from build123d import *

# Parameters (mm, degrees)
SKETCH1_W           = 196
SKETCH1_H           = 90
BOSS_EXTRUDE1_DEPTH = 55
SKETCH2_W           = 45.25
SKETCH2_H           = 40.5
SKETCH2_H_2         = 84
CUT_EXTRUDE1_DEPTH  = 52


with BuildPart() as part:
    # Sketch1 → Boss-Extrude1 (new body)
    with BuildSketch(Plane(origin=(0, 0, 0), x_dir=(1, 0, 0), z_dir=(0, 1, 0))):
        Rectangle(SKETCH1_W, SKETCH1_H)
    extrude(amount=BOSS_EXTRUDE1_DEPTH)

    # Sketch2 → Cut-Extrude1 (cut)
    with BuildSketch(Plane(origin=(0, 55, 0), x_dir=(1, 0, 0), z_dir=(0, 1, 0))):
        with Locations((-72.375, 21.75)):
            Rectangle(SKETCH2_W, SKETCH2_H)
        with Locations((-72.375, -21.75)):
            Rectangle(SKETCH2_W, SKETCH2_H)
        with Locations((-24.125, 21.75)):
            Rectangle(SKETCH2_W, SKETCH2_H)
        with Locations((-24.125, -21.75)):
            Rectangle(SKETCH2_W, SKETCH2_H)
        with Locations((24.125, 21.75)):
            Rectangle(SKETCH2_W, SKETCH2_H)
        with Locations((24.125, -21.75)):
            Rectangle(SKETCH2_W, SKETCH2_H)
        with Locations((72.375, 0)):
            Rectangle(SKETCH2_W, SKETCH2_H_2)
    extrude(amount=-CUT_EXTRUDE1_DEPTH, mode=Mode.SUBTRACT)


solid = part.part
The model under review builds one solid part; all positions refer to its coordinate system, in mm. Round coordinates to 2 decimals unless told otherwise and drop trailing zeros. Write each loop counter-clockwise with the first axis right and the second up, starting at its lowest first coordinate (ties: lowest second). Pieces come first, ordered by that corner, then holes. Notation, with made-up numbers: (73, 47) - (82, 47) arc R23 ccw to (82, 64) - close; hole circle Ø5 at (7.25, 23). An arc over 180 degrees is marked (long way). One line per item, written item: value. Start each with the question number.
1. Consider section C-C on z = 38. Write out the cut boundary in (x, y), and give its area (3 significant figures).
2. Consider section D-D on x = 60.5. Write out the cut boundary in (y, z).
3. Consider section A-A on y = 30.5. State how many separate pieces and enclosed holes the cut face has, and give its area (3 significant figures).
4. To check wall thickness, follow L1, parallel to X at y = 35, z = -38; L2, parallel to Z at x = -89, y = 30; L3, parallel to Z at x = 51.5, y = 10. State the ranges of each line that lie inside material, in increasing order. Write a range as from..to.
5. Consider section B-B on x = -67.5. Write out the cut boundary in (y, z).
6. Clearance check with flat-ended pins moving along their axes: P1, Ø2, axis at x = 9.5, z = 11.5, coming from the +Y side; P2, Ø10, axis at x = 59.5, z = -13, coming from the -Y side. State where each tip first meets the part, or that it passes through.
Checks:
1. outline: (-98, 0) - (98, 0) - (98, 55) - (95, 55) - (95, 3) - (49.75, 3) - (49.75, 55) - (46.75, 55) - (46.75, 3) - (1.5, 3) - (1.5, 55) - (-1.5, 55) - (-1.5, 3) - (-46.75, 3) - (-46.75, 55) - (-49.75, 55) - (-49.75, 3) - (-95, 3) - (-95, 55) - (-98, 55) - close
1. area: 1,370 mm^2
2. outline: (0, -45) - (55, -45) - (55, -42) - (3, -42) - (3, 42) - (55, 42) - (55, 45) - (0, 45) - close
3. separate pieces: 1
3. enclosed holes: 7
3. area: 2,840 mm^2
4. L1: x = -98..-95, -49.75..-46.75, -1.5..1.5, 46.75..49.75, 95..98
4. L2: z = -45..-42, -1.5..1.5, 42..45
4. L3: z = -45..-42, 42..45
5. outline: (0, -45) - (55, -45) - (55, -42) - (3, -42) - (3, -1.5) - (55, -1.5) - (55, 1.5) - (3, 1.5) - (3, 42) - (55, 42) - (55, 45) - (0, 45) - close
6. P1: stops at y = 3
6. P2: stops at y = 0
